Check sheet for the drawn part. Datum: minimum x, y, z corner. Units: mm. A direction names the side the tool comes from. Give positions to 0.01 mm unless a question says otherwise; leave off trailing zeros. Order: outer loops, then holes, each group sorted by start corner. A loop starts at its lowest first (then second) coordinate and runs counter-clockwise, first axis right, second up. Notation, with made-up numbers: (49.5, 14) -> (105.5, 14) arc R31 cw to (105.5, 48) -> close; hole circle Ø1 at (58.25, -18). An arc over 180 degrees is marked (long way). Return JSON: item names as keys, results as strings. Group by question number.
(1) Release check for a two-part mould opening along X. For the marked faces 5, 6 and 7 record: pulls with the +X half, pulls with the -X half, needs draft (parallel to the pull), parting line crosses it, or undercut.
(2) Tool access check on the marked faces 1, 2, 3 and 4. Record the directions out of +Z, -Z, +X, -X, +Y, -Y that give a thin tool (end or side, any length) a straight path to the whole face; none if there is none.
(3) Depth check by flat-ended pin: pin 1 Ø2.5 at (y, z) = (10, 3) entering from +X; pin 2 Ø0.5 at (x, z) = (52.5, 8.5) entering from -Y; pin 3 Ø5 at (x, y) = (70, 9.775) entering from +Z; pin 4 Ø10 at (x, y) = (61.5, 17.5) entering from +Z. Enter the tip coordinate at first touch or a pass-through.
(4) Cross-section at A-A on x = 70. Enter the section's corners in (y, z) (3 decimals), then the cut area to 4 significant figures.
(5) Thickness scan on line 1 along Y through (x, z) = (56.5, 3); line 2 along Y through (x, z) = (70, 1.05) (3 decimals); line 3 along X through (y, z) = (10, 7.75). Record the ranges inside material, lowest first.
(6) Cross-section at C-C on x = 12. Enter the section's corners in (y, z), then the cut area to 4 significant figures.
(7) Cross-section at B-B on z = 6.5. State how many separate pieces and enclosed holes the cut face has, then the cut area to 3 significant figures.
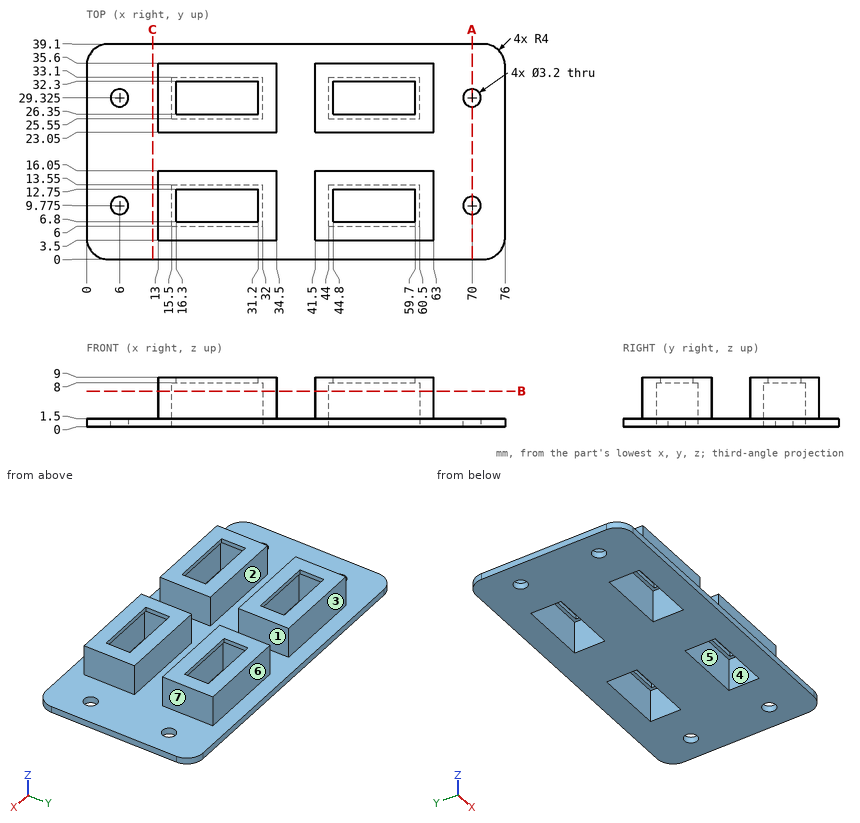
Verdict:
{
 "1": {"face 5": "undercut", "face 6": "needs draft", "face 7": "pulls with the +X half"},
 "2": {"face 1": "+Z, +Y, -Y", "face 2": "+Z, +X, -X", "face 3": "+Z, +X, -X, +Y", "face 4": "-Z"},
 "3": {"pin 1": "x = 63", "pin 2": "y = 3.5", "pin 3": "z = 1.5", "pin 4": "z = 9"},
 "4": {"outline": "(0, 0) -> (8.175, 0) -> (8.175, 1.5) -> (0, 1.5) -> close; (11.375, 0) -> (27.725, 0) -> (27.725, 1.5) -> (11.375, 1.5) -> close; (30.925, 0) -> (39.1, 0) -> (39.1, 1.5) -> (30.925, 1.5) -> close", "area": "49.05 mm²"},
 "5": {"line 1": "3.5 to 6, 13.55 to 16.05, 23.05 to 25.55, 33.1 to 35.6", "line 2": "0 to 8.175, 11.375 to 27.725, 30.925 to 39.1", "line 3": "13 to 15.5, 32 to 34.5, 41.5 to 44, 60.5 to 63"},
 "6": {"outline": "(0, 0) -> (39.1, 0) -> (39.1, 1.5) -> (0, 1.5) -> close", "area": "58.65 mm²"},
 "7": {"separate pieces": "4", "enclosed holes": "4", "area": "581 mm²"}
}
